Geometry: final body of the model. Coordinates: model frame, mm. Face numbers are marked on the shaded views. A direction names the side the tool comes from. Round coordinates to 2 decimals unless told otherwise and drop trailing zeros. Loops run counter-clockwise (first coordinate to the right, second up) from the corner with the lowest first, then second, coordinate; pieces in that order, holes last. Notation, with made-up numbers: (71.25, -21.5) - (105.25, -21.5) arc R18 cw to (105.25, -12.5) - close; hole circle Ø2 at (74.5, 46). An arc over 180 degrees is marked (long way). Write item = value, one per line. Start each with the question number.
Item 1: Access query for the marked faces 1 and 2. Directions: +Z, -Z, +X, -X, +Y, -Y. A direction counts if a zero-diameter tool reaches every point of the face in a straight line with its end or side. Return the directions, or none.
Item 2: Section B-B (x = 208). Return loops of the section in (y, z), plus the area to 3 significant figures.
Item 3: Section A-A (y = -12). Return loops of the section in (x, z), plus the area to 3 significant figures.
Item 4: Line query: line 1 (Z direction, x = 75, y = -42); line 2 (Z direction, x = -256.5, y = 26.5); line 3 (X direction, y = 0, z = -20). Output: solid intervals per line, ascending. Write a range as from..to.
Item 5: First-contact query: pin 1 (3 mm diameter, centred on y = -62, z = -22.5, fed in from -X); pin 2 (10 mm diameter, centred on y = -40.5, z = -33.5, fed in from -X); pin 3 (1.5 mm diameter, centred on y = -86, z = -36, fed in from -X). Flat tips, straight axial feed; report the tip coordinate or a pass-through.
Item 6: Draft query along Z for the marked faces 3, 4 and 5. Return one class per face: pulls with the +Z half, pulls with the -Z half, needs draft (parallel to the pull), parting line crosses it, or undercut.
Item 7: Section C-C (z = 12). Return loops of the section in (x, y), plus the area to 3 significant figures.
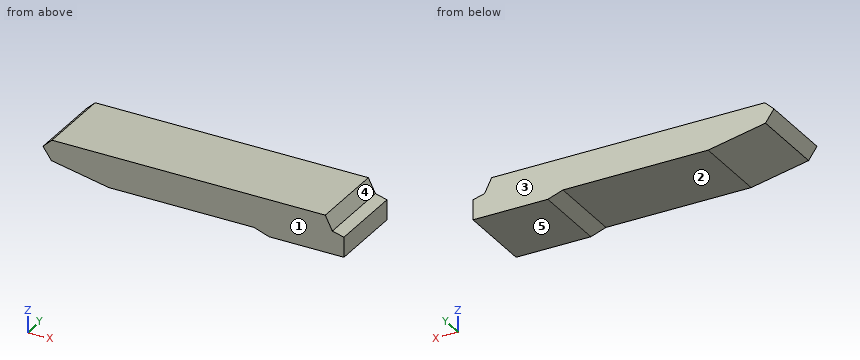
Autodesk Inventor part; units mm, degrees
ref_plane "YZ Plane" through (0, 0, 0) normal (1, 0, 0) x (0, 1, 0)
ref_plane "XZ Plane" through (0, 0, 0) normal (0, 1, 0) x (-1, 0, 0)
ref_plane "XY Plane" through (0, 0, 0) normal (0, 0, 1) x (1, 0, 0)
sketch "Sketch1" plane through (0, 0, 0) normal (0, 1, 0) x (-1, 0, 0)
  line L0 (364.2, 20.66) -> (392.2, -5.97)
  line L1 (392.2, -5.97) -> (366, -43.36)
  line L2 (366, -43.36) -> (187.3, -78.36)
  line L3 (187.3, -78.36) -> (-264.9, -78.36)
  line L4 (-264.9, -78.36) -> (-311.9, -94.56)
  line L5 (-311.9, -94.56) -> (-544.9, -94.56)
  line L6 (-544.9, -94.56) -> (-544.9, -32.16)
  line L7 (-544.9, -32.16) -> (-508.9, -22.77)
  line L8 (-508.9, -22.77) -> (-486.9, 20.66)
  line L9 (364.2, 20.66) -> (-486.9, 20.66)
  point P0 (0, 0)
  dimension "d0" = 20.66
  dimension "d1" = 5.97
  dimension "d2" = 43.36
  dimension "d3" = 78.36
  dimension "d4" = 78.36
  dimension "d5" = 94.56
  dimension "d6" = 94.56
  dimension "d7" = 32.16
  dimension "d8" = 22.77
  dimension "d9" = 20.66
  dimension "d10" = 364.2
  dimension "d11" = 392.2
  dimension "d12" = 366
  dimension "d13" = 187.3
  dimension "d14" = 264.9
  dimension "d15" = 311.9
  dimension "d16" = 544.9
  dimension "d17" = 544.9
  dimension "d18" = 508.9
  dimension "d19" = 486.9
extrude "Extrusion1" add sketch "Sketch1" along normal mid plane 238.9
properties part number "Friend_hull_collision"
Taken from the geometry:
q1.face_1 = +Z, -Z, +X, -X, -Y
q1.face_2 = -Z, -X, +Y, -Y
q2.outline = (-119.45, -78.36) - (119.45, -78.36) - (119.45, 20.66) - (-119.45, 20.66) - close
q2.area = 23,700 mm^2
q3.outline = (-392.2, -5.97) - (-366, -43.36) - (-187.3, -78.36) - (264.9, -78.36) - (311.9, -94.56) - (544.9, -94.56) - (544.9, -32.16) - (508.9, -22.77) - (486.9, 20.66) - (-364.2, 20.66) - close
q3.area = 89,800 mm^2
q4.line_1 = -78.36..20.66
q4.line_2 = -64.81..20.66
q4.line_3 = -382.37..507.5
q5.pin_1 = -381.67
q5.pin_2 = -376.41
q5.pin_3 = -371.68
q6.face_3 = needs draft
q6.face_4 = pulls with the +Z half
q6.face_5 = pulls with the -Z half
q7.outline = (-373.31, -119.45) - (491.29, -119.45) - (491.29, 119.45) - (-373.31, 119.45) - close
q7.area = 207,000 mm^2
